The model under review builds one solid part; all positions refer to its coordinate system, in mm. Face numbers are marked on the shaded views. Round coordinates to 2 decimals unless told otherwise and drop trailing zeros. Write each loop counter-clockwise with the first axis right and the second up, starting at its lowest first coordinate (ties: lowest second). Pieces come first, ordered by that corner, then holes. Notation, with made-up numbers: M -21.75,79 L 30.25,79 A20 ccw 30.25,104 Z; hole C -17,-32.5 d2. An arc over 180 degrees is marked long. Write item = value, one per line. Start each with the question number.
Item 1: Take a section at C-C, the plane y = 32.5. Give the boundary of the cut face in (x, z), plus the area to 3 significant figures.
Item 2: Take a section at D-D, the plane y = 3.5. Give the boundary of the cut face in (x, z).
Item 3: Take a section at B-B, the plane z = 0. Give the boundary of the cut face in (x, y), plus the area to 3 significant figures.
Item 4: Take a section at A-A, the plane x = 0. Give the boundary of the cut face in (y, z).
Item 5: The part is to be moulded in two halves that separate along X. For the marked faces 1, 2 and 3, say which applies: +X half, -X half, draft (parallel to the pull), parting line (faces both ways), or undercut.
Item 6: To check wall thickness, follow line 1 along Y through (x, z) = (10, 5.5); line 2 along X through (y, z) = (14, 0); line 3 along X through (y, z) = (8.5, 0). State the ranges of each line that lie inside material, in increasing order.
Item 7: For pin 1 Ø5 at (y, z) = (24.5, -22.5) entering from +X; pin 2 Ø1 at (x, y) = (-1, 37.5) entering from -Z; pin 3 Ø10 at (x, y) = (-16, 34) entering from +Z, all flat-tipped, find the tip position at first contact; note any pin that passes through.
from build123d import *

# Parameters (mm, degrees)
CUT_EXTRUDE1_DEPTH      = 63.261545114
CUT_EXTRUDE1_DEPTH_BACK = 63.261545114
SKETCH3_R               = 5
CUT_EXTRUDE2_DEPTH      = 63.060454569
CUT_EXTRUDE2_DEPTH_BACK = 63.060454569
SKETCH4_R               = 5


with BuildPart() as part:
    # Sketch2 → Revolve1 (revolve)
    with BuildSketch(Plane.XY, mode=Mode.PRIVATE) as revolve1_sk:
        Polygon((11.25, 0), (22.5, 0), (32.5, 42), (26.332276244, 42), (19.189419101, 12), (11.25, 12), align=None)
    revolve(revolve1_sk.sketch.rotate(Axis((0, 0, 0), (0, 1, 0)), 90), axis=Axis((0, 0, 0), (0, 1, 0)))

    # Sketch3 → Cut-Extrude1 (cut, two sides: drawn at the far end of the back side and taken through both)
    with BuildSketch(Plane(origin=(0, 0, 0), x_dir=(0, 0, -1), z_dir=(1, 0, 0)).offset(-CUT_EXTRUDE1_DEPTH_BACK)):
        with Locations((0, 42)):
            Circle(SKETCH3_R)
    extrude(amount=CUT_EXTRUDE1_DEPTH + CUT_EXTRUDE1_DEPTH_BACK, mode=Mode.SUBTRACT)

    # Sketch4 → Cut-Extrude2 (cut, two sides: drawn at the far end of the back side and taken through both)
    with BuildSketch(Plane.XY.offset(-CUT_EXTRUDE2_DEPTH_BACK)):
        with Locations((0, 42)):
            Circle(SKETCH4_R)
    extrude(amount=CUT_EXTRUDE2_DEPTH + CUT_EXTRUDE2_DEPTH_BACK, mode=Mode.SUBTRACT)


solid = part.part
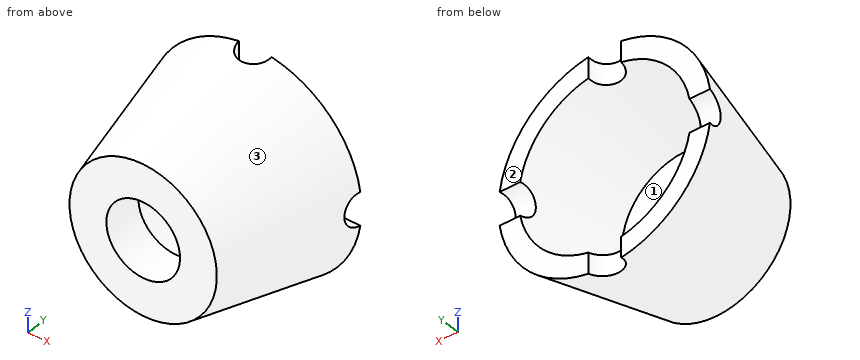
Response values:
q1.outline = C 0,0 d60.48; hole C 0,0 d48.14
q1.area = 1,050 mm2
q2.outline = C 0,0 d46.67; hole C 0,0 d22.5
q3.outline = M -31.31,37 L -22.5,0 L -11.25,0 L -11.25,12 L -19.19,12 L -25.14,37 Z; M 11.25,0 L 22.5,0 L 31.31,37 L 25.14,37 L 19.19,12 L 11.25,12 Z
q3.area = 613 mm2
q4.outline = M 0,-22.5 L 37,-31.31 L 37,-25.14 L 12,-19.19 L 12,-11.25 L 0,-11.25 Z; M 0,11.25 L 12,11.25 L 12,19.19 L 37,25.14 L 37,31.31 L 0,22.5 Z
q5.face_1 = undercut
q5.face_2 = draft
q5.face_3 = parting line
q6.line_1 = 0 to 12
q6.line_2 = -25.83 to -19.67, 19.67 to 25.83
q6.line_3 = -24.52 to -11.25, 11.25 to 24.52
q7.pin_1 = 20.21
q7.pin_2 = -31.33
q7.pin_3 = 28.93
